Check sheet for the modelled part. Datum: model origin and axes. Units: mm. A direction names the side the tool comes from. Coordinates: 2 decimals unless noted, no trailing zeros. Write each loop counter-clockwise with the first axis right and the second up, starting at its lowest first coordinate (ties: lowest second). Pieces come first, ordered by that corner, then holes. Notation, with made-up numbers: M -34.75,67 L -30.75,67 A21 ccw -30.75,106 Z; hole C 3.25,89.25 d10. An arc over 180 degrees is marked long. Answer as CSV lines item,"result". Start each with the question number.
Q1. Sectioned sample at A-A, the plane z = 0. Record the cut outline in (x, y), then the cut area to 3 significant figures.
Q2. Mould release check, pull along Y, two halves, no side actions. Record for faces 1 (the cylindrical face through (1.88, 21.23, 5.96)), 2 (the cylindrical face through (-0.07, 2.496, 0.065)), 3 (the flat face through (0, 0, 0)): pulls with the +Y half, pulls with the -Y half, needs draft (parallel to the pull), parting line crosses it, or undercut.
Q3. Thickness scan on line 1 along Y through (x, z) = (1, 0); line 2 along Y through (x, z) = (-4.5, 4); line 3 along Z through (x, y) = (-2, 2). Record the ranges inside material, lowest first. Write a range as from..to.
Q4. Sectioned sample at B-B, the plane x = 0. Record the cut outline in (y, z), then the cut area to 3 significant figures.
Q5. Depth check by flat-ended pin: pin 1 Ø1 at (x, y) = (2.5, 16.5) entering from +Z; pin 2 Ø2 at (x, y) = (-5, 5) entering from +Z; pin 3 Ø3 at (x, y) = (0.5, 8) entering from -Z. Enter the tip coordinate at first touch or a pass-through.
Q6. Sectioned sample at C-C, the plane z = -2.25. Record the cut outline in (x, y).
Q7. Access from +Z, -Z, +X, -X, +Y, -Y to the whole of each face (thin tool, end or side, straight path). Record for faces 4 (the cylindrical face through (-4.88, 9.86, -1.08)), 5 (the flat face through (0, 22.5, 0)).
Q8. Sectioned sample at D-D, the plane y = 2.75. Record the cut outline in (x, z), then the cut area to 3 significant figures.
from build123d import *

# Parameters (mm, degrees)
SKETCH1_R               = 5
BOSS_EXTRUDE1_DEPTH     = 20
SKETCH3_R               = 6.25
BOSS_EXTRUDE3_DEPTH     = 2.5
CUT_EXTRUDE1_DEPTH      = 25.173849507
CUT_EXTRUDE1_DEPTH_BACK = 25.173849507
SKETCH4_R               = 0.5


with BuildPart() as part:
    # Sketch1 → Boss-Extrude1 (new body)
    with BuildSketch(Plane(origin=(0, 0, 0), x_dir=(1, 0, 0), z_dir=(0, 1, 0))):
        with Locations(Location((0, 0, 0), (0, 0, 270))):
            Circle(SKETCH1_R)
    extrude(amount=BOSS_EXTRUDE1_DEPTH)

    # Sketch3 → Boss-Extrude3 (add)
    with BuildSketch(Plane(origin=(0, 20, 0), x_dir=(1, 0, 0), z_dir=(0, 1, 0))):
        with Locations(Location((0, 0, 0), (0, 0, 270))):
            Circle(SKETCH3_R)
    extrude(amount=BOSS_EXTRUDE3_DEPTH)

    # Sketch4 → Cut-Extrude1 (cut, two sides: drawn at the far end of the back side and taken through both)
    with BuildSketch(Plane(origin=(0, 0, 0), x_dir=(0, 0, -1), z_dir=(1, 0, 0)).offset(-CUT_EXTRUDE1_DEPTH_BACK)):
        with Locations((0, 2)):
            Circle(SKETCH4_R)
    extrude(amount=CUT_EXTRUDE1_DEPTH + CUT_EXTRUDE1_DEPTH_BACK, mode=Mode.SUBTRACT)


solid = part.part
Output:
1,outline,"M -6.25,20 L -5,20 L -5,2.5 L 5,2.5 L 5,20 L 6.25,20 L 6.25,22.5 L -6.25,22.5 Z; M -5,0 L 5,0 L 5,1.5 L -5,1.5 Z"
1,area,"221 mm^2"
2,face 1,"needs draft"
2,face 2,"undercut"
2,face 3,"pulls with the -Y half"
3,line 1,"y = 0..1.5, 2.5..22.5"
3,line 2,"y = 20..22.5"
3,line 3,"z = -4.58..-0.5, 0.5..4.58"
4,outline,"M 0,-5 L 20,-5 L 20,-6.25 L 22.5,-6.25 L 22.5,6.25 L 20,6.25 L 20,5 L 0,5 Z; hole C 2,0 d1"
4,area,"230 mm^2"
5,pin 1,"stops at z = 4.58"
5,pin 2,"stops at z = 3"
5,pin 3,"stops at z = -5"
6,outline,"M -5.83,20 L -4.47,20 L -4.47,0 L 4.47,0 L 4.47,20 L 5.83,20 L 5.83,22.5 L -5.83,22.5 Z"
7,face 4,"-Y"
7,face 5,"+Z, -Z, +X, -X, +Y"
8,outline,"C 0,0 d10"
8,area,"78.5 mm^2"
